For this review, use the dimensioned drawing (mm, ordinates from the lowest corner) and the shaded views. A direction names the side the tool comes from. Coordinates: 2 decimals unless noted, no trailing zeros. Loops run counter-clockwise (first coordinate to the right, second up) from the corner with the lowest first, then second, coordinate; pieces in that order, holes last. Notation, with made-up numbers: (84, 22.25) -> (120, 22.25) arc R32 ccw to (120, 60.25) -> close; hole circle Ø5 at (-30, 78). An arc over 180 degrees is marked (long way). One line per question, with ' | ' between items. Start each with the question number.
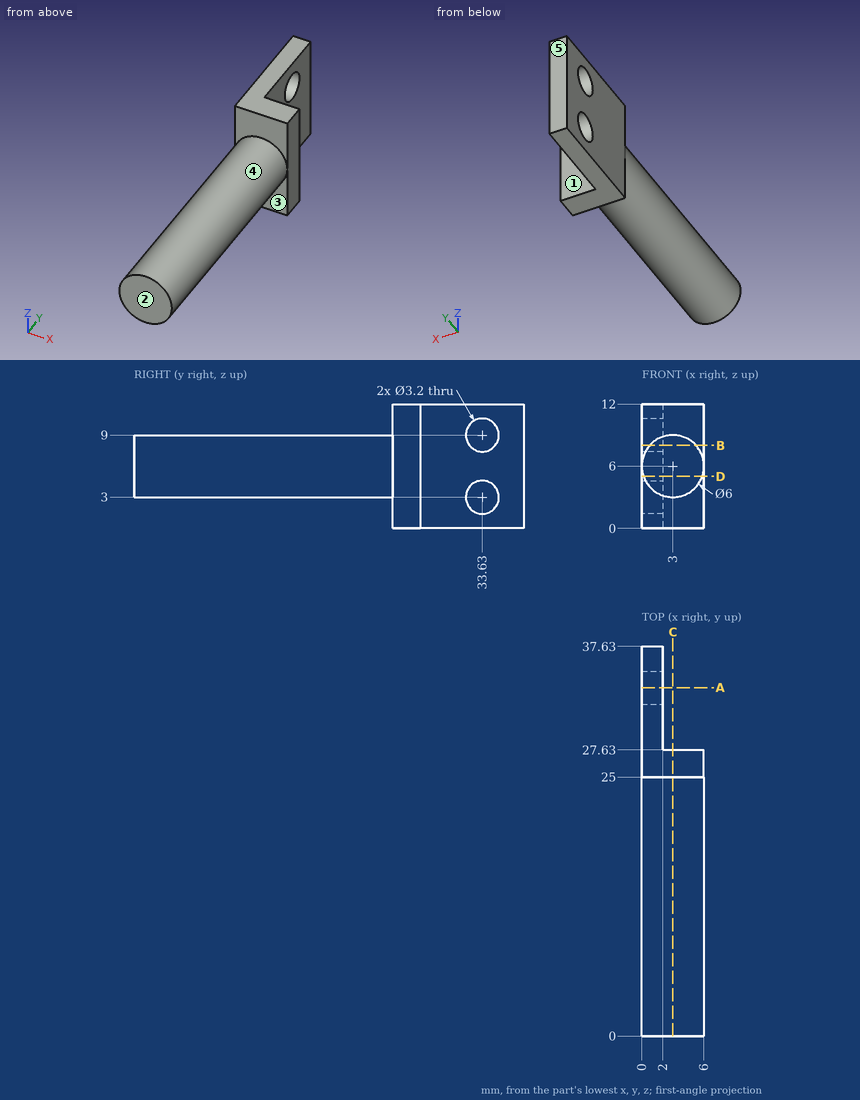
1) Consider section D-D, the plane z = 5. Write out the cut boundary in (x, y).
2) Machinability: for the marked faces 1, 2, 3, 4 and 5, which of the approach directions +Z, -Z, +X, -X, +Y, -Y give a long, thin tool a straight path to every point of the face, cutting with its end or side? Answer none if there is none.
3) Consider section C-C, the plane x = 3. Write out the cut boundary in (y, z).
4) Consider section A-A, the plane y = 33.63. Write out the cut boundary in (x, z), plus the area to 3 significant figures.
5) Consider section B-B, the plane z = 8. Write out the cut boundary in (x, y), plus the area to 3 significant figures.
6) Wall thickness on L1, parallel to Z at x = 1.4, y = 33.63; L2, parallel to Y at x = 1.35, z = 3; L3, parallel to Y at x = 4, z = 2.25: over which ranges is each line inside the solid? List them lowest first.
7) Insertion check: pin 1 Ø1.8 at (x, z) = (3, 8) entering from -Y; pin 2 Ø3 at (x, z) = (4, 6.5) entering from +Y; pin 3 Ø3 at (y, z) = (31.5, 4.5) entering from +X. Each pin has a flat end and moves straight along its axis. Give the tip position at first contact, or say it passes through.
Filled sheet:
1) outline: (0, 25) -> (0.17, 25) -> (0.17, 0) -> (5.83, 0) -> (5.83, 25) -> (6, 25) -> (6, 27.63) -> (2, 27.63) -> (2, 37.63) -> (0, 37.63) -> close
2) face 1: +Z, -Z, +X, +Y | face 2: +Z, -Z, +X, -X, -Y | face 3: -Z, -Y | face 4: -Y | face 5: +Z, -Z, +X, -X, +Y
3) outline: (0, 3) -> (25, 3) -> (25, 0) -> (27.63, 0) -> (27.63, 12) -> (25, 12) -> (25, 9) -> (0, 9) -> close
4) outline: (0, 0) -> (2, 0) -> (2, 1.4) -> (0, 1.4) -> close; (0, 4.6) -> (2, 4.6) -> (2, 7.4) -> (0, 7.4) -> close; (0, 10.6) -> (2, 10.6) -> (2, 12) -> (0, 12) -> close | area: 11.2 mm^2
5) outline: (0, 25) -> (0.76, 25) -> (0.76, 0) -> (5.24, 0) -> (5.24, 25) -> (6, 25) -> (6, 27.63) -> (2, 27.63) -> (2, 32.38) -> (0, 32.38) -> close; (0, 34.88) -> (2, 34.88) -> (2, 37.63) -> (0, 37.63) -> close | area: 143 mm^2
6) L1: 0 to 1.4, 4.6 to 7.4, 10.6 to 12 | L2: 25 to 32.03, 35.23 to 37.63 | L3: 25 to 27.63
7) pin 1: y = 0 | pin 2: y = 27.63 | pin 3: x = 2
